The listing builds one solid part. Answer for the finished solid, in the listing's coordinates (mm). A direction names the side the tool comes from. Round coordinates to 2 decimals unless told otherwise and drop trailing zeros. Order: outer loops, then holes, each group sorted by start corner. A loop starts at its lowest first (then second) coordinate and runs counter-clockwise, first axis right, second up. Notation, with made-up numbers: (-7, -15.5) - (40, -15.5) arc R15 ccw to (40, 6.5) - close; hole circle Ø11 at (83, 24). An arc over 180 degrees is marked (long way). One line per item, written item: value. Start each with the question number.
1. Section C-C, the plane x = 11 is taken. Give the vertices of the cut face in (y, z).
2. Straight lines are drawn through the part: line 1 (Z direction, x = 7.5, y = 14); line 2 (Z direction, x = 8, y = 1); line 3 (Z direction, x = -6, y = -2). For each, find the intervals that lie inside material, in ascending order.
3. Section D-D, the plane y = 19.5 is taken. Give the vertices of the cut face in (x, z), then the cut area to 3 significant figures.
4. For a pull along Z with two mould halves and no side action, classify faces 3 (the flat face through (0, -4, 0)), 4 (the cylindrical face through (5, 0, 20)), 5 (the cylindrical face through (0, -12, -1)) as released by +Z, released by -Z, zero draft, split by the parting line, or undercut.
5. Section A-A, the plane y = -16 is taken. Give the vertices of the cut face in (x, z).
6. Flat-ended cylindrical pins translate along their axes: P1, Ø8, axis at y = -2, z = 7, coming from the +X side; P2, Ø6, axis at x = 13, z = 7, coming from the -Y side; P3, Ø3.5, axis at x = -1, y = -6.5, coming from the -Z side; P4, Ø0.5, axis at x = 0, z = -0.5, coming from the +Y side. Find the tip coordinate at first contact, or state that the pin passes through.
7. Section B-B, the plane z = 39.5 is taken. Give the vertices of the cut face in (x, y), then the cut area to 3 significant figures.
8. A tool of negligible diameter and unlimited length cuts with its end or side. For faces 1 (the flat face through (0.3, 0.3, -2)), 2 (the flat face through (-12.08, 8.085, -0.986)), from which of +Z, -Z, +X, -X, +Y, -Y can it reach the whole face along a straight path? Write none if from no direction.
from build123d import *

# Parameters (mm, degrees)
SKETCH1_R           = 25
BOSS_EXTRUDE1_DEPTH = 5
SKETCH2_RX          = 2.1
SKETCH2_RY          = 1.5
SKETCH2_R           = 0.518128849
BOSS_EXTRUDE2_DEPTH = 2
SKETCH3_R           = 0.5
CUT_EXTRUDE1_DEPTH  = 36.707142143
BOSS_EXTRUDE4_START = 2
SKETCH4_R           = 25
SKETCH4_R_2         = 23.007381087
BOSS_EXTRUDE4_DEPTH = 2


with BuildPart() as part:
    # Sketch1 → Boss-Extrude1 (new body)
    with BuildSketch(Plane.XY):
        Circle(SKETCH1_R)
    extrude(amount=BOSS_EXTRUDE1_DEPTH)

    # Sketch2 → Boss-Extrude2 (add)
    # profile 1 of 5: a face of its own
    with BuildSketch(Plane(origin=(0, 0, 0), x_dir=(-1, 0, 0), z_dir=(0, 0, -1))):
        with BuildLine():
            Line((14.136829803, 0.416245401), (15.569591433, 8.79462198))
            ThreePointArc((15.569591433, 8.79462198), (18.762283071, 11.116793185), (14.997353799, 9.928909953))
            Line((14.997353799, 9.928909953), (9.08074084, 6.188095723))
            Line((9.08074084, 6.188095723), (9.08074084, 4.188095723))
            ThreePointArc((9.08074084, 4.188095723), (5.390688396, 8.422617088), (0, 10))
            ThreePointArc((0, 10), (-5.390688396, 8.422617088), (-9.08074084, 4.188095723))
            Line((-9.08074084, 4.188095723), (-9.08074084, 6.188095723))
            Line((-9.08074084, 6.188095723), (-14.997353799, 9.928909953))
            ThreePointArc((-14.997353799, 9.928909953), (-18.762283071, 11.116793185), (-15.569591433, 8.79462198))
            Line((-15.569591433, 8.79462198), (-14.136829803, 0.416245401))
            Line((-14.136829803, 0.416245401), (-11.971082941, -0.83257025))
            ThreePointArc((-11.971082941, -0.83257025), (0, -12), (11.971082941, -0.83257025))
            Line((11.971082941, -0.83257025), (14.136829803, 0.416245401))
        make_face()
        with BuildLine():
            Line((-0.758529186, 1.832589074), (-0.758529186, 2.393390515))
            ThreePointArc((-0.758529186, 2.393390515), (0, 6.13651388), (0.758529186, 2.393390515))
            Line((0.758529186, 2.393390515), (0.758529186, 1.832589074))
            Line((0.758529186, 1.832589074), (-0.758529186, 1.832589074))
        make_face(mode=Mode.SUBTRACT)
        with BuildLine():
            ThreePointArc((-6.236314399, 1.832589074), (0, -10.485460932), (6.236314399, 1.832589074))
            Line((6.236314399, 1.832589074), (0, 0))
            Line((0, 0), (-6.236314399, 1.832589074))
        make_face(mode=Mode.SUBTRACT)
    # profile 2 of 5: a face of its own
    with BuildSketch(Plane(origin=(0, 0, 0), x_dir=(-1, 0, 0), z_dir=(0, 0, -1))):
        with Locations(Location((-3.116282157, -3.288657736), (0, 0, -90))):
            Ellipse(SKETCH2_RX, SKETCH2_RY)
    # profile 3 of 5: a face of its own
    with BuildSketch(Plane(origin=(0, 0, 0), x_dir=(-1, 0, 0), z_dir=(0, 0, -1))):
        with Locations(Location((3.116282157, -3.288657736), (0, 0, -90))):
            Ellipse(SKETCH2_RX, SKETCH2_RY)
    # profile 4 of 5: a face of its own
    with BuildSketch(Plane(origin=(0, 0, 0), x_dir=(-1, 0, 0), z_dir=(0, 0, -1))):
        with Locations((0.878678891, 4.497077937)):
            Circle(SKETCH2_R)
    # profile 5 of 5: a face of its own
    with BuildSketch(Plane(origin=(0, 0, 0), x_dir=(-1, 0, 0), z_dir=(0, 0, -1))):
        with Locations(Location((-0.878678891, 4.497077937, 0), (0, 0, 180))):
            Circle(SKETCH2_R)
    extrude(amount=BOSS_EXTRUDE2_DEPTH)

    # Sketch3 → Cut-Extrude1 (cut, through all)
    with BuildSketch(Plane(origin=(0, 0, 0), x_dir=(-1, 0, 0), z_dir=(0, 0, -1))):
        with Locations((9.782386324, 12.497076735)):
            Circle(SKETCH3_R)
        with Locations((9.782386324, 15.910239984)):
            Circle(SKETCH3_R)
        with Locations((9.782386324, 9.13143185)):
            Circle(SKETCH3_R)
        with Locations((4.501388335, 12.497076735)):
            Circle(SKETCH3_R)
        with Locations((4.501388335, 15.910239984)):
            Circle(SKETCH3_R)
        with Locations((9.782386324, -17.768118771)):
            Circle(SKETCH3_R)
        with Locations((9.783740136, -13.926982269)):
            Circle(SKETCH3_R)
        with Locations((9.713673566, -10.704966648)):
            Circle(SKETCH3_R)
        with Locations((4.501388335, -17.768118771)):
            Circle(SKETCH3_R)
        with Locations((4.501388335, -13.810006537)):
            Circle(SKETCH3_R)
        with Locations((-4.501388335, 15.910239984)):
            Circle(SKETCH3_R)
        with Locations((-4.501388335, 12.497076735)):
            Circle(SKETCH3_R)
        with Locations((-9.782386324, 12.497076735)):
            Circle(SKETCH3_R)
        with Locations((-9.782386324, 15.910239984)):
            Circle(SKETCH3_R)
        with Locations((-9.782386324, 9.13143185)):
            Circle(SKETCH3_R)
        with Locations((-4.501388335, -17.768118771)):
            Circle(SKETCH3_R)
        with Locations((-4.501388335, -13.810006537)):
            Circle(SKETCH3_R)
        with Locations((-9.783740136, -13.926982269)):
            Circle(SKETCH3_R)
        with Locations((-9.713673566, -10.704966648)):
            Circle(SKETCH3_R)
        with Locations((-9.782386324, -17.768118771)):
            Circle(SKETCH3_R)
    extrude(amount=-CUT_EXTRUDE1_DEPTH, mode=Mode.SUBTRACT)

    # Sketch4 → Boss-Extrude4 (add)
    with BuildSketch(Plane(origin=(0, 0, 0), x_dir=(-1, 0, 0), z_dir=(0, 0, -1)).offset(BOSS_EXTRUDE4_START)):
        Circle(SKETCH4_R)
        Circle(SKETCH4_R_2, mode=Mode.SUBTRACT)
    extrude(amount=-BOSS_EXTRUDE4_DEPTH)

    # Sketch5 → Revolve1 (revolve)
    with BuildSketch(Plane(origin=(0, 0, 0), x_dir=(0, 0, -1), z_dir=(1, 0, 0)), mode=Mode.PRIVATE) as revolve1_sk:
        with BuildLine():
            Line((-5, 5), (-35, 5))
            Line((-35, 5), (-35, 8))
            ThreePointArc((-35, 8), (-35.585786438, 9.414213562), (-37, 10))
            Line((-37, 10), (-43, 10))
            ThreePointArc((-43, 10), (-44.414213562, 9.414213562), (-45, 8))
            Line((-45, 8), (-45, 0))
            Line((-45, 0), (-5, 0))
            Line((-5, 0), (-5, 5))
        make_face()
    revolve(revolve1_sk.sketch.rotate(Axis((0, 0, 0), (0, 0, 1)), 90), axis=Axis((0, 0, 0), (0, 0, 1)))


solid = part.part
Answer list:
1. outline: (-22.45, -2) - (-20.21, -2) - (-20.21, 0) - (-4.8, 0) - (-4.8, -2) - (7.4, -2) - (7.4, 0) - (20.21, 0) - (20.21, -2) - (22.45, -2) - (22.45, 5) - (-22.45, 5) - close
2. line 1: z = 0 to 5
2. line 2: z = -2 to 5, 35 to 45
2. line 3: z = 0 to 5, 35 to 45
3. outline: (-15.64, -2) - (-12.21, -2) - (-12.21, 0) - (12.21, 0) - (12.21, -2) - (15.64, -2) - (15.64, 5) - (-15.64, 5) - close
3. area: 170 mm²
4. face 3: released by -Z
4. face 4: undercut
4. face 5: zero draft
5. outline: (-19.21, -2) - (-16.53, -2) - (-16.53, 0) - (16.53, 0) - (16.53, -2) - (19.21, -2) - (19.21, 5) - (-19.21, 5) - close
6. P1: stops at x = 25
6. P2: stops at y = -22.56
6. P3: stops at z = 0
6. P4: stops at y = 25
7. outline: circle Ø20 at (0, 0)
7. area: 314 mm²
8. face 1: -Z, +X, -X, +Y, -Y
8. face 2: -Z
